Read the model definition and answer for the solid it produces. Units are mm, in the model's axes. Face numbers are marked on the shaded views. Give positions to 0.01 mm unless a question says otherwise; leave off trailing zeros. Order: outer loops, then holes, each group sorted by start corner. A loop starts at its lowest first (then second) coordinate and runs counter-clockwise, first axis right, second up. Notation, with made-up numbers: (-35.75, -24.75) - (17.25, -24.75) arc R10 cw to (17.25, -14.75) - close; hole circle Ø10 at (-11, -1). An arc over 180 degrees is marked (long way). Write item = value, one per line.
```python
from build123d import *

# Parameters (mm, degrees)
F0_W     = 66.04
F0_H     = 30.48
F0_W_2   = 61.7728
F0_H_2   = 26.416
F1_DEPTH = 23.3934
F2_DEPTH = 26.2382
F3_W     = 18.8468
F3_H     = 2.8448
F4_DEPTH = 4.445
F5_W     = 18.8468
F5_H     = 2.8448
F6_DEPTH = 4.445


with BuildPart() as f1:
    # F0 (on Top) → F1 (new body)
    with BuildSketch(Plane.XY):
        with Locations((5.729598, -1.061104)):
            Rectangle(F0_W, F0_H)
        with Locations((5.729598, -1.061104)):
            Rectangle(F0_W_2, F0_H_2, mode=Mode.SUBTRACT)
    extrude(amount=F1_DEPTH)

    # F0 (on Top) → F2 (join)
    with BuildSketch(Plane.XY):
        with Locations((5.729598, -1.061104)):
            Rectangle(F0_W_2, F0_H_2)
    extrude(amount=F2_DEPTH)

    # F3 (on face) → F4 (cut)
    with BuildSketch(Plane.XZ.offset(14.269104)):
        with Locations((1.259198, 24.8158)):
            Rectangle(F3_W, F3_H)
    extrude(amount=-F4_DEPTH, mode=Mode.SUBTRACT)

    # F5 (on face) → F6 (cut)
    with BuildSketch(Plane(origin=(0, 12.146896, 0), x_dir=(-1, 0, 0), z_dir=(0, 1, 0))):
        with Locations((-1.767198, 24.8158)):
            Rectangle(F5_W, F5_H)
    extrude(amount=-F6_DEPTH, mode=Mode.SUBTRACT)


solid = f1.part
```
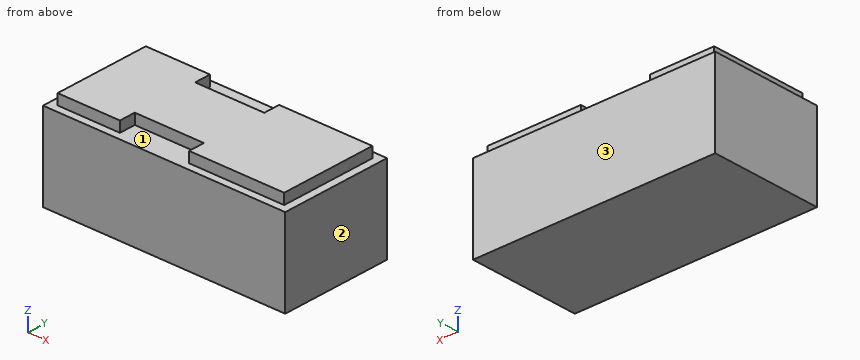
1. Flat-ended cylindrical pins translate along their axes: pin 1 (1.4 mm diameter, centred on y = -11.5, z = 24.5, fed in from +X); pin 2 (1.4 mm diameter, centred on x = -20, z = 25, fed in from -Y); pin 3 (2.5 mm diameter, centred on x = 2.5, z = 25, fed in from -Y). Find the tip coordinate at first contact, or state that the pin passes through.
Recorded:
pin_1 = 36.62
pin_2 = -14.27
pin_3 = -9.82
2. Straight lines are drawn through the part: L1, parallel to X at y = -13, z = 24; L2, parallel to X at y = -2.5, z = 24; L3, parallel to Z at x = 8, y = 9.5. For each, find the intervals that lie inside material, in ascending order. Write a range as [from, to].
Recorded:
L1 = [-25.16, -8.16], [10.68, 36.62]
L2 = [-25.16, 36.62]
L3 = [0, 23.39]
3. Determine the mould class of the marked faces 1, 2 and 3 for opening direction X: +X half, -X half, draft (parallel to the pull), parting line (faces both ways), or undercut.
Recorded:
face_1 = undercut
face_2 = +X half
face_3 = draft
4. Section B-B (x = 5) is taken. Determine the outline of the cut face in (y, z).
Recorded:
outline = (-16.3, 0) - (14.18, 0) - (14.18, 23.39) - (7.7, 23.39) - (7.7, 26.24) - (-9.82, 26.24) - (-9.82, 23.39) - (-16.3, 23.39) - close
5. Section A-A (y = -13.5) is taken. Determine the outline of the cut face in (x, z).
Recorded:
outline = (-27.29, 0) - (38.75, 0) - (38.75, 23.39) - (36.62, 23.39) - (36.62, 26.24) - (10.68, 26.24) - (10.68, 23.39) - (-8.16, 23.39) - (-8.16, 26.24) - (-25.16, 26.24) - (-25.16, 23.39) - (-27.29, 23.39) - close
